from build123d import *

# Parameters (mm, degrees)
SKETCH1_R           = 1.5
BOSS_EXTRUDE3_DEPTH = 3.85


with BuildPart() as part:
    # Sketch1 → Boss-Extrude3 (new body, symmetric)
    with BuildSketch(Plane(origin=(0, 0, 0), x_dir=(1, 0, 0), z_dir=(0, 1, 0))):
        with BuildLine():
            Line((-13.75, -15), (0, -15))
            Line((0, -15), (0, 0))
            Line((0, 0), (2, 0))
            Line((2, 0), (2, 30))
            Line((2, 30), (-1, 30))
            ThreePointArc((-1, 30), (-1.576352013, 29.869367868), (-2.040057994, 29.503003078))
            Line((-2.040057994, 29.503003078), (-11.530466398, 17.748937838))
            ThreePointArc((-11.530466398, 17.748937838), (-13.178803317, 14.798188939), (-13.75, 11.466872681))
            Line((-13.75, 11.466872681), (-13.75, -15))
        make_face()
        with Locations((-10.75, -12)):
            Circle(SKETCH1_R, mode=Mode.SUBTRACT)
        with Locations((-3, -12)):
            Circle(SKETCH1_R, mode=Mode.SUBTRACT)
    extrude(amount=BOSS_EXTRUDE3_DEPTH, both=True)


solid = part.part
Could you check a few things on this model? Use its own coordinates, in mm. A direction names the side the tool comes from. Round coordinates to 2 decimals unless told otherwise and drop trailing zeros. Write each loop counter-clockwise with the first axis right and the second up, starting at its lowest first coordinate (ties: lowest second). Pieces come first, ordered by that corner, then holes. Notation, with made-up numbers: (84.25, 80) -> (99.25, 80) arc R14 cw to (99.25, 88) -> close; hole circle Ø7 at (31, -27). An arc over 180 degrees is marked (long way). Use a Markdown table: item, result.
1. We'd pull the mould along Z, two halves only. Please class faces 3 (the face through (-1.614, -0.054, 12.575)), 4 (the face through (-12.25, -0.05, 11.93)), 5 (the face through (-6.719, 0.054, -23.708)), 6 (the face through (0, 0, 8)): +Z half, -Z half, draft (parallel to the pull), parting line (faces both ways), or undercut.
Answer key:
| item | result |
|---|---|
| face 3 | undercut |
| face 4 | undercut |
| face 5 | -Z half |
| face 6 | draft |
2. If we section it at B-B (y = -2.25): List the corners of the cut face in (x, z) for me.
Answer key:
| item | result |
|---|---|
| outline | (-13.75, -11.47) arc R10 ccw to (-11.53, -17.75) -> (-2.04, -29.5) arc R1.34 ccw to (-1, -30) -> (2, -30) -> (2, 0) -> (0, 0) -> (0, 15) -> (-13.75, 15) -> close; hole circle Ø3 at (-10.75, 12); hole circle Ø3 at (-3, 12) |
3. If we section it at A-A (z = 12): List the corners of the cut face in (x, y) for me, then the cut area to 3 significant figures.
Answer key:
| item | result |
|---|---|
| outline | (-13.75, -3.85) -> (-12.25, -3.85) -> (-12.25, 3.85) -> (-13.75, 3.85) -> close; (-9.25, -3.85) -> (-4.5, -3.85) -> (-4.5, 3.85) -> (-9.25, 3.85) -> close; (-1.5, -3.85) -> (0, -3.85) -> (0, 3.85) -> (-1.5, 3.85) -> close |
| area | 59.7 mm^2 |
4. For pin 1 Ø4 at (y, z) = (-2.5, 2.5) entering from +X; pin 2 Ø3 at (x, y) = (-8.5, -3) entering from -Z; pin 3 Ø2 at (x, y) = (1.5, 0) entering from +Z, each with a flat end and sliding along its axis, tell me the tip position at first contact or that it passes through.
Answer key:
| item | result |
|---|---|
| pin 1 | stops at x = 0 |
| pin 2 | stops at z = -23.36 |
| pin 3 | stops at z = 0 |
5. If we section it at D-D (z = 7): List the corners of the cut face in (x, y) for me.
Answer key:
| item | result |
|---|---|
| outline | (-13.75, -3.85) -> (0, -3.85) -> (0, 3.85) -> (-13.75, 3.85) -> close |
6. Please list where these lines run through material, in increasing order: probe 1 along X at (y, z) = (-0.5, 12); probe 2 along X at (y, z) = (-3, 12.5); probe 3 along X at (y, z) = (-2.5, 8).
Answer key:
| item | result |
|---|---|
| probe 1 | x = -13.75 to -12.25, -9.25 to -4.5, -1.5 to 0 |
| probe 2 | x = -13.75 to -12.16, -9.34 to -4.41, -1.59 to 0 |
| probe 3 | x = -13.75 to 0 |
7. If we section it at C-C (x = -10.75): List the corners of the cut face in (y, z) for me, then the cut area to 3 significant figures.
Answer key:
| item | result |
|---|---|
| outline | (-3.85, -18.72) -> (3.85, -18.72) -> (3.85, 10.5) -> (-3.85, 10.5) -> close; (-3.85, 13.5) -> (3.85, 13.5) -> (3.85, 15) -> (-3.85, 15) -> close |
| area | 237 mm^2 |
8. Which directions (+Z, -Z, +X, -X, +Y, -Y) give clear straight access to the entire face, cutting with the end or side of a thin tool? Please do faces 1 (the face through (1, 0, -30)), 2 (the face through (1, 0, 0)).
Answer key:
| item | result |
|---|---|
| face 1 | -Z, +X, -X, +Y, -Y |
| face 2 | +Z, +X, +Y, -Y |
